Check sheet for the modelled part. Datum: model origin and axes. Units: mm. A direction names the side the tool comes from. Round coordinates to 2 decimals unless told otherwise and drop trailing zeros. Order: outer loops, then holes, each group sorted by start corner. A loop starts at its lowest first (then second) coordinate and runs counter-clockwise, first axis right, second up.
(1) Depth check by flat-ended pin: pin 1 (16 mm diameter, centred on x = -57.5, y = 23, fed in from +Z). Enter the tip coordinate at first touch or a pass-through.
(2) Sectioned sample at A-A, the plane z = 38. Enter the section's corners in (x, y) (3 decimals), and give its area (3 significant figures).
(3) Sectioned sample at B-B, the plane x = 46.5. Enter the section's corners in (y, z) (3 decimals).
(4) Tool access check on faces 1 (the flat face through (-1, 1, 0)), 2 (the flat face through (66.675, -26, 38)). Record the directions out of +Z, -Z, +X, -X, +Y, -Y that give a thin tool (end or side, any length) a straight path to the whole face; none if there is none.
(5) Mould release check, pull along Y, two halves, no side actions. Record for faces 3 (the flat face through (-76.2, -1, 25)), 4 (the flat face through (51, 41.275, 38)), 5 (the flat face through (-51, -25, 25.4)): released by +Y, released by -Y, zero draft, split by the parting line, or undercut.
(6) Sectioned sample at C-C, the plane y = -30. Enter the section's corners in (x, z) (3 decimals), and give its area (3 significant figures).
(7) Thickness scan on probe 1 along X at (y, z) = (-26.5, 26.5) (3 decimals); probe 2 along Y at (x, z) = (15, 47) (3 decimals); probe 3 along Z at (x, y) = (58, 16.5). Record the ranges inside material, lowest first.
```python
from build123d import *

# Parameters (mm, degrees)
F0_W     = 152.4
F0_H     = 101.6
F0_W_2   = 31.75
F0_H_2   = 31.75
F1_DEPTH = 50.8
F2_DEPTH = 25.4


with BuildPart() as f1:
    # F0 (on Top) → F1 (new body)
    with BuildSketch(Plane.XY):
        Rectangle(F0_W, F0_H)
        with Locations((-50.8, -25.4)):
            Rectangle(F0_W_2, F0_H_2, mode=Mode.SUBTRACT)
        Polygon((-15.875, -9.525), (0, -9.525), (15.875, -9.525), (15.875, -41.275), (-15.875, -41.275), align=None, mode=Mode.SUBTRACT)
        with Locations((50.8, -25.4)):
            Rectangle(F0_W_2, F0_H_2, mode=Mode.SUBTRACT)
        with Locations((-50.8, 25.4)):
            Rectangle(F0_W_2, F0_H_2, mode=Mode.SUBTRACT)
        Polygon((-15.875, 9.525), (-15.875, 41.275), (15.875, 41.275), (15.875, 9.525), (0, 9.525), align=None, mode=Mode.SUBTRACT)
        with Locations((50.8, 25.4)):
            Rectangle(F0_W_2, F0_H_2, mode=Mode.SUBTRACT)
    extrude(amount=F1_DEPTH)

    # F0 (on Top) → F2 (join)
    with BuildSketch(Plane.XY):
        with Locations((-50.8, 25.4)):
            Rectangle(F0_W_2, F0_H_2)
        Polygon((15.875, 41.275), (-15.875, 41.275), (-15.875, 9.525), (0, 9.525), (15.875, 9.525), align=None)
        with Locations((50.8, 25.4)):
            Rectangle(F0_W_2, F0_H_2)
        with Locations((50.8, -25.4)):
            Rectangle(F0_W_2, F0_H_2)
        Polygon((15.875, -9.525), (0, -9.525), (-15.875, -9.525), (-15.875, -41.275), (15.875, -41.275), align=None)
        with Locations((-50.8, -25.4)):
            Rectangle(F0_W_2, F0_H_2)
    extrude(amount=F2_DEPTH)


solid = f1.part
```
Derived:
1. pin 1: stops at z = 25.4
2. outline: (-76.2, -50.8) - (76.2, -50.8) - (76.2, 50.8) - (-76.2, 50.8) - close; hole (-66.675, -41.275) - (-34.925, -41.275) - (-34.925, -9.525) - (-66.675, -9.525) - close; hole (-66.675, 9.525) - (-34.925, 9.525) - (-34.925, 41.275) - (-66.675, 41.275) - close; hole (-15.875, -41.275) - (15.875, -41.275) - (15.875, -9.525) - (-15.875, -9.525) - close; hole (-15.875, 9.525) - (15.875, 9.525) - (15.875, 41.275) - (-15.875, 41.275) - close; hole (34.925, -41.275) - (66.675, -41.275) - (66.675, -9.525) - (34.925, -9.525) - close; hole (34.925, 9.525) - (66.675, 9.525) - (66.675, 41.275) - (34.925, 41.275) - close
2. area: 9,440 mm2
3. outline: (-50.8, 0) - (50.8, 0) - (50.8, 50.8) - (41.275, 50.8) - (41.275, 25.4) - (9.525, 25.4) - (9.525, 50.8) - (-9.525, 50.8) - (-9.525, 25.4) - (-41.275, 25.4) - (-41.275, 50.8) - (-50.8, 50.8) - close
4. face 1: -Z, +X, -X, +Y, -Y
4. face 2: +Z
5. face 3: zero draft
5. face 4: undercut
5. face 5: undercut
6. outline: (-76.2, 0) - (76.2, 0) - (76.2, 50.8) - (66.675, 50.8) - (66.675, 25.4) - (34.925, 25.4) - (34.925, 50.8) - (15.875, 50.8) - (15.875, 25.4) - (-15.875, 25.4) - (-15.875, 50.8) - (-34.925, 50.8) - (-34.925, 25.4) - (-66.675, 25.4) - (-66.675, 50.8) - (-76.2, 50.8) - close
6. area: 5,320 mm2
7. probe 1: x = -76.2 to -66.675, -34.925 to -15.875, 15.875 to 34.925, 66.675 to 76.2
7. probe 2: y = -50.8 to -41.275, -9.525 to 9.525, 41.275 to 50.8
7. probe 3: z = 0 to 25.4
